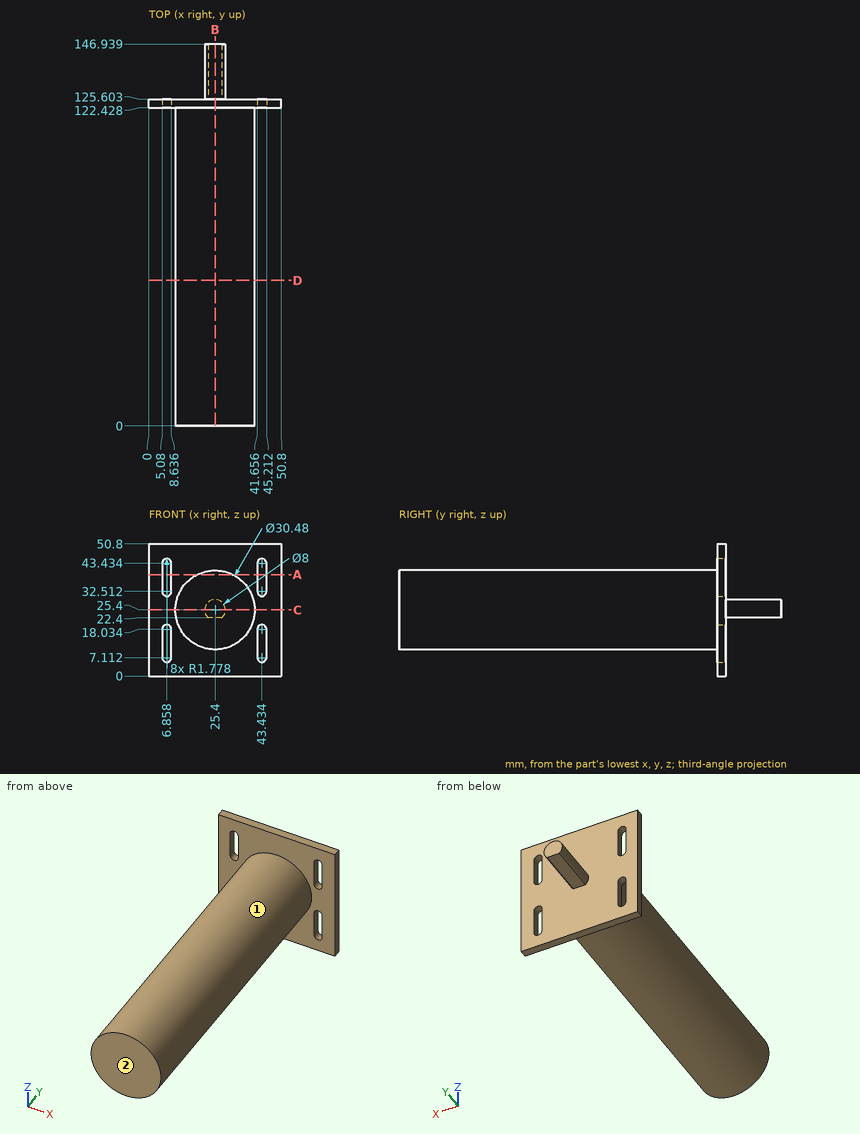
For this review, use the dimensioned drawing (mm, ordinates from the lowest corner) and the shaded views. A direction names the side the tool comes from. Coordinates: 2 decimals unless noted, no trailing zeros. Loops run counter-clockwise (first coordinate to the right, second up) from the corner with the lowest first, then second, coordinate; pieces in that order, holes last. Notation, with made-up numbers: (5.25, -24.5) -> (25.25, -24.5) arc R25 ccw to (25.25, -6.5) -> close; hole circle Ø2 at (-29.5, 36). An arc over 180 degrees is marked (long way). Return JSON: item names as keys, results as strings. Group by question number.
(1) Consider section A-A, the plane z = 39. Give the boundary of the cut face in (x, y).
(2) For pin 1 Ø1.5 at (y, z) = (75, 34.5) entering from -X; pin 2 Ø6 at (x, y) = (26, 135) entering from -Z; pin 3 Ø4 at (x, z) = (43, 26) entering from +Y, all flat-tipped, find the tip position at first contact; note any pin that passes through.
(3) Consider section B-B, the plane x = 25.4. Give the boundary of the cut face in (y, z), plus the area to 3 significant figures.
(4) Consider section C-C, the plane z = 25.4. Give the boundary of the cut face in (x, y), plus the area to 3 significant figures.
(5) Tool access review of the marked faces 1 and 2: name each direction out of +Z, -Z, +X, -X, +Y, -Y from which nothing blocks a thin tool from reaching the whole face with its end or side.
(6) To check wall thickness, follow L1, parallel to Y at x = 13, z = 18; L2, parallel to Y at x = 47, z = 4; L3, parallel to Z at x = 34, y = 92. State the ranges of each line that lie inside material, in increasing order.
(7) Consider section D-D, the plane y = 56. Give the boundary of the cut face in (x, z).
Results below:
{
 "1": {"outline": "(0, 122.43) -> (5.08, 122.43) -> (5.08, 125.6) -> (0, 125.6) -> close; (8.64, 122.43) -> (18.52, 122.43) -> (18.52, 0) -> (32.28, 0) -> (32.28, 122.43) -> (41.66, 122.43) -> (41.66, 125.6) -> (8.64, 125.6) -> close; (45.21, 122.43) -> (50.8, 122.43) -> (50.8, 125.6) -> (45.21, 125.6) -> close"},
 "2": {"pin 1": "stops at x = 12.65", "pin 2": "stops at z = 22.4", "pin 3": "stops at y = 125.6"},
 "3": {"outline": "(0, 10.16) -> (122.43, 10.16) -> (122.43, 0) -> (125.6, 0) -> (125.6, 22.4) -> (146.94, 22.4) -> (146.94, 29.4) -> (125.6, 29.4) -> (125.6, 50.8) -> (122.43, 50.8) -> (122.43, 40.64) -> (0, 40.64) -> close", "area": "4,040 mm2"},
 "4": {"outline": "(0, 122.43) -> (10.16, 122.43) -> (10.16, 0) -> (40.64, 0) -> (40.64, 122.43) -> (50.8, 122.43) -> (50.8, 125.6) -> (29.4, 125.6) -> (29.4, 146.94) -> (21.4, 146.94) -> (21.4, 125.6) -> (0, 125.6) -> close", "area": "4,060 mm2"},
 "5": {"face 1": "-Y", "face 2": "+Z, -Z, +X, -X, -Y"},
 "6": {"L1": "y = 0 to 125.6", "L2": "y = 122.43 to 125.6", "L3": "z = 12.82 to 37.98"},
 "7": {"outline": "circle Ø30.48 at (25.4, 25.4)"}
}
